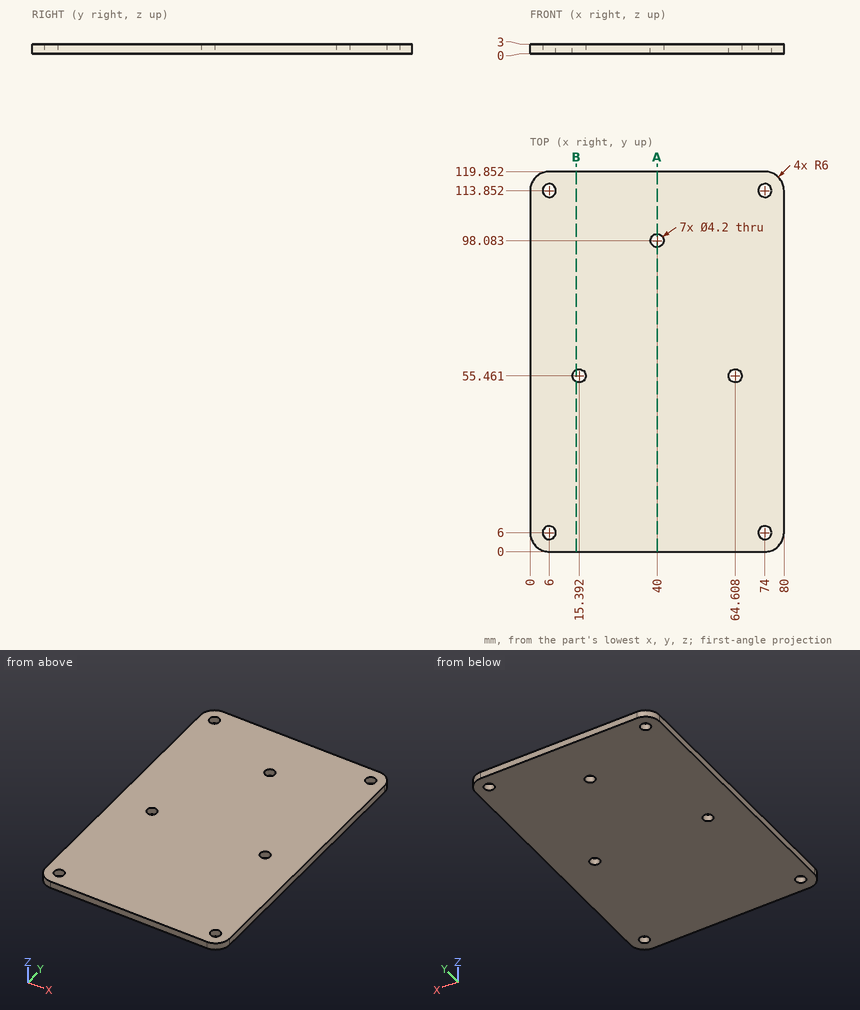
Job drawing, mm, ordinate dimensions from the low corner. One solid piece. Round coordinates to 2 decimals unless told otherwise and drop trailing zeros. Loops run counter-clockwise (first coordinate to the right, second up) from the corner with the lowest first, then second, coordinate; pieces in that order, holes last.
Item 1: Cut at B-B, the plane x = 14.5. Give the cut face in (y, z).
Item 2: Cut at A-A, the plane x = 40. Give the cut face in (y, z).
Item 3: Drill centre lines: line 1 (Y direction, x = 6, z = 0.9); line 2 (Y direction, x = 40, z = 1.9); line 3 (Y direction, x = 74.5, z = 0.4). Where is each one in solid material? Low to high.
A:
1. outline: (0, 0) - (53.56, 0) - (53.56, 3) - (0, 3) - close; (57.36, 0) - (119.85, 0) - (119.85, 3) - (57.36, 3) - close
2. outline: (0, 0) - (95.98, 0) - (95.98, 3) - (0, 3) - close; (100.18, 0) - (119.85, 0) - (119.85, 3) - (100.18, 3) - close
3. line 1: y = 0 to 3.9, 8.1 to 111.75, 115.95 to 119.85
3. line 2: y = 0 to 95.98, 100.18 to 119.85
3. line 3: y = 0.02 to 3.96, 8.04 to 111.81, 115.89 to 119.83
